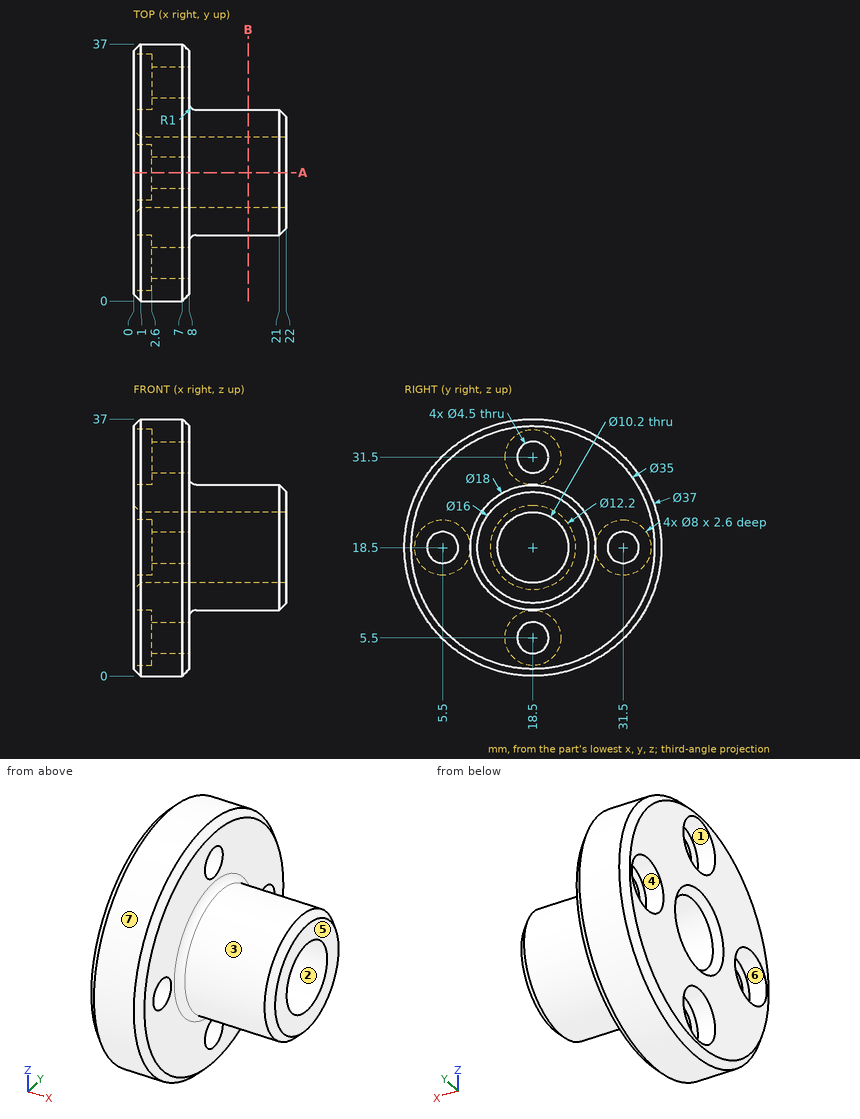
Could you check a few things on this drawing? It's one solid part, dimensions in mm from its lowest x, y, z. A direction names the side the tool comes from. Round coordinates to 2 decimals unless told otherwise and drop trailing zeros. Write each loop counter-clockwise with the first axis right and the second up, starting at its lowest first coordinate (ties: lowest second). Pieces come first, ordered by that corner, then holes. Notation, with made-up numbers: (-35, 13) -> (2, 13) arc R16 ccw to (2, 20) -> close; hole circle Ø7 at (29, -21.75). An arc over 180 degrees is marked (long way). One line per item, written item: value.
1) For the marked faces 1, 2 and 3, which set-ups out of +Z, -Z, +X, -X, +Y, -Y let a thin tool reach every point of the face, with its end or its side?
Filled sheet:
face 1: -X
face 2: +X, -X
face 3: +X
2) If I drill on line 1 (Y direction, x = 5.1, z = 18.5); line 2 (X direction, y = 12, z = 29); line 3 (Z direction, x = 1.9, y = 5.5), over which ranges is the centre line in solid material (lowest first)? Write a range as [from, to].
Filled sheet:
line 1: y = [0, 3.25], [7.75, 13.4], [23.6, 29.25], [33.75, 37]
line 2: x = [0, 8]
line 3: z = [5.34, 14.5], [22.5, 31.66]
3) Suppose I cut it at B-B on x = 16.5. List the corners of the cut face in (y, z) for me, plus the area to 3 significant figures.
Filled sheet:
outline: circle Ø18 at (18.5, 18.5); hole circle Ø10.2 at (18.5, 18.5)
area: 173 mm2
4) We'd pull the mould along Y, two halves only. Please class the marked faces 4, 5, 6 and 7: released by +Y, released by -Y, zero draft, split by the parting line, or undercut.
Filled sheet:
face 4: undercut
face 5: zero draft
face 6: undercut
face 7: split by the parting line
5) I'm going to push flat-ended pins straight in: pin 1 Ø6 at (x, z) = (18, 24) entering from +Y; pin 2 Ø6.5 at (y, z) = (31.5, 18.5) entering from -X; pin 3 Ø9 at (y, z) = (18.5, 31.5) entering from +X. Where does each tip first touch, or does it pass through?
Filled sheet:
pin 1: stops at y = 27.15
pin 2: stops at x = 2.6
pin 3: stops at x = 21.5
6) Suppose I cut it at A-A on y = 18.5. Give the number of separate pieces and of enclosed holes in the cut face, plus the area to 3 significant figures.
Filled sheet:
separate pieces: 4
enclosed holes: 0
area: 230 mm2
